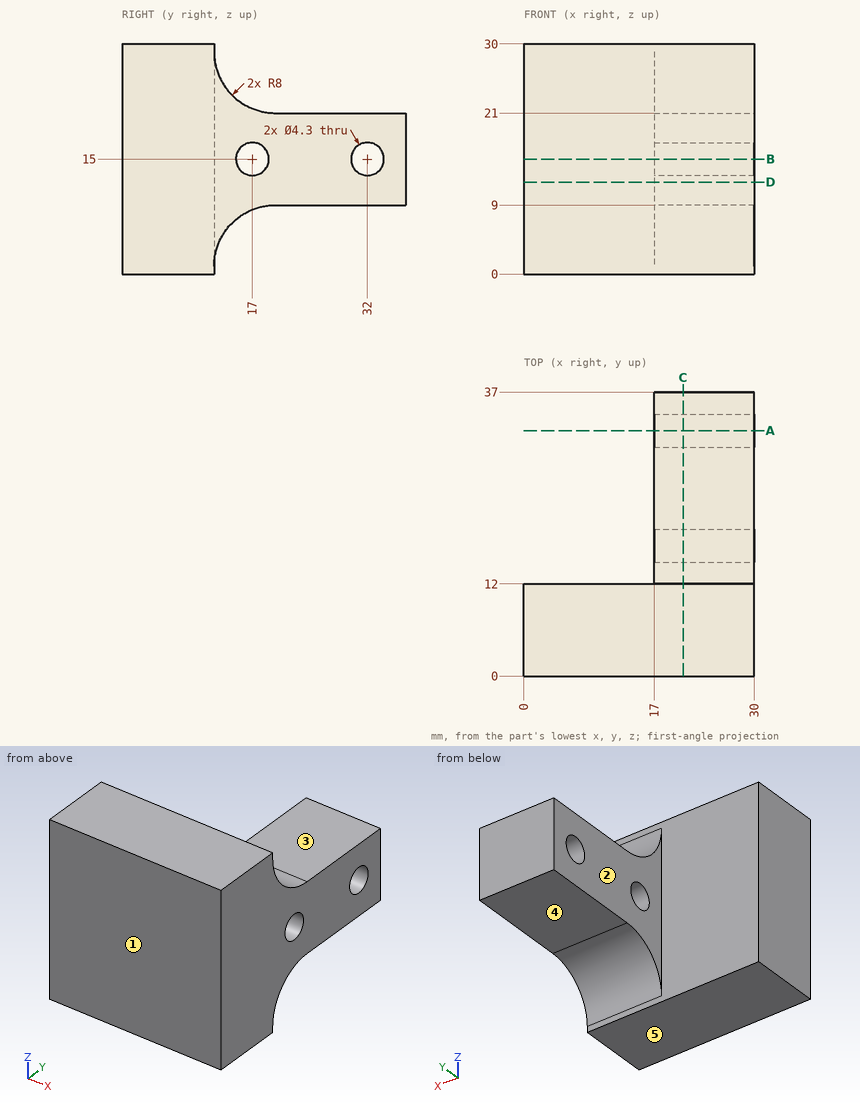
Study the drawing (mm; zero at the part's minimum x, y, z) and answer. A direction names the side the tool comes from. Give positions to 0.01 mm unless a question says otherwise; leave off trailing zeros. Order: outer loops, then holes, each group sorted by start corner. A loop starts at its lowest first (then second) coordinate and runs counter-clockwise, first axis right, second up. Notation, with made-up numbers: M 14.25,-26 L 64.25,-26 A21 ccw 64.25,13 Z; hole C 28.25,-16 d6. An arc over 180 degrees is marked long. Put each result on its own line as item: value. Start each with the question number.
Item 1: The part is cut by section B-B, the plane z = 15. Determine the outline of the cut face in (x, y).
Item 2: Which of the six approach directions +Z, -Z, +X, -X, +Y, -Y give full straight-line access (tool end or side, diameter ignored) to the marked faces 1, 2, 3, 4 and 5?
Item 3: The part is cut by section A-A, the plane y = 32. Determine the outline of the cut face in (x, z).
Item 4: The part is cut by section D-D, the plane z = 12. Determine the outline of the cut face in (x, y).
Item 5: Flat-ended cylindrical pins translate along their axes: P1, Ø14.5, axis at x = 26.5, y = 27, coming from the +Z side; P2, Ø4, axis at x = 26.5, y = 17, coming from the +Z side (3 decimals); P3, Ø4, axis at x = 24.5, y = 32.5, coming from the -Z side. Find the tip coordinate at first contact, or state that the pin passes through.
Item 6: The part is cut by section C-C, the plane x = 20.75. Determine the outline of the cut face in (y, z).
Item 7: Find the intervals of material crossed by line 1 along Y through (x, z) = (22.25, 15); line 2 along Z through (x, y) = (27, 27); line 3 along Y through (x, z) = (11.25, 20), in increasing order.
Answer key:
1. outline: M 0,0 L 30,0 L 30,14.85 L 17,14.85 L 17,12 L 0,12 Z; M 17,19.15 L 30,19.15 L 30,29.85 L 17,29.85 Z; M 17,34.15 L 30,34.15 L 30,37 L 17,37 Z
2. face 1: +Z, -Z, +X, -X, -Y
2. face 2: +Z, -Z, -X, +Y
2. face 3: +Z, +X, -X, +Y
2. face 4: -Z, +X, -X, +Y
2. face 5: -Z, +X, -X, +Y, -Y
3. outline: M 17,9 L 30,9 L 30,12.85 L 17,12.85 Z; M 17,17.15 L 30,17.15 L 30,21 L 17,21 Z
4. outline: M 0,0 L 30,0 L 30,37 L 17,37 L 17,12 L 0,12 Z
5. P1: stops at z = 21
5. P2: stops at z = 22.755
5. P3: stops at z = 9
6. outline: M 0,0 L 12,0 L 12,1 A8 cw 20,9 L 37,9 L 37,21 L 20,21 A8 cw 12,29 L 12,30 L 0,30 Z; hole C 17,15 d4.3; hole C 32,15 d4.3
7. line 1: y = 0 to 14.85, 19.15 to 29.85, 34.15 to 37
7. line 2: z = 9 to 21
7. line 3: y = 0 to 12
